```python
from build123d import *

# Parameters (mm, degrees)
BOSS_EXTRUDE1_DEPTH = 2.2
SKETCH2_W           = 9
SKETCH2_H           = 2.2
SKETCH2_W_2         = 42.2
BOSS_EXTRUDE2_DEPTH = 22.8
SKETCH3_W           = 9
SKETCH3_H           = 2.2
CUT_EXTRUDE1_DEPTH  = 50.796084183
SKETCH4_R           = 1.5
CUT_EXTRUDE2_DEPTH  = 54.851740919
SKETCH5_R           = 4
SKETCH5_R_2         = 1.5
CUT_EXTRUDE3_DEPTH  = 53.866340899


with BuildPart() as part:
    # Sketch1 → Boss-Extrude1 (new body)
    with BuildSketch(Plane(origin=(0, 0, 0), x_dir=(1, 0, 0), z_dir=(0, 1, 0))):
        Polygon((21.1, 0), (-21.1, 0), (-21.1, 8), (-30.1, 8), (-30.1, 33), (-21.1, 33), (-21.1, 27), (-18.1, 27), (-18.1, 37), (18.1, 37), (18.1, 27), (21.1, 27), (21.1, 33), (30.1, 33), (30.1, 8), (21.1, 8), align=None)
    extrude(amount=BOSS_EXTRUDE1_DEPTH)

    # Sketch2 → Boss-Extrude2 (add)
    with BuildSketch(Plane(origin=(0, 2.2, 0), x_dir=(1, 0, 0), z_dir=(0, 1, 0))):
        with Locations((25.6, 31.9)):
            Rectangle(SKETCH2_W, SKETCH2_H)
        with Locations((-25.6, 31.9)):
            Rectangle(SKETCH2_W, SKETCH2_H)
        with Locations((0, 1.1)):
            Rectangle(SKETCH2_W_2, SKETCH2_H)
    extrude(amount=BOSS_EXTRUDE2_DEPTH)

    # Sketch3 → Cut-Extrude1 (cut, through all)
    with BuildSketch(Plane.XY.offset(-30.8)):
        with Locations((-25.6, 23.9)):
            Rectangle(SKETCH3_W, SKETCH3_H)
    extrude(amount=-CUT_EXTRUDE1_DEPTH, mode=Mode.SUBTRACT)

    # Sketch4 → Cut-Extrude2 (cut, through all)
    with BuildSketch(Plane.XY):
        with Locations((-17.5, 13)):
            Circle(SKETCH4_R)
        with Locations((-10.5, 13)):
            Circle(SKETCH4_R)
        with Locations((-10.5, 20)):
            Circle(SKETCH4_R)
        with Locations((-3.5, 13)):
            Circle(SKETCH4_R)
        with Locations((-10.5, 6)):
            Circle(SKETCH4_R)
        with Locations((10.5, 6)):
            Circle(SKETCH4_R)
        with Locations((3.5, 13)):
            Circle(SKETCH4_R)
        with Locations((10.5, 20)):
            Circle(SKETCH4_R)
        with Locations((10.5, 13)):
            Circle(SKETCH4_R)
        with Locations((17.5, 13)):
            Circle(SKETCH4_R)
    extrude(amount=-CUT_EXTRUDE2_DEPTH, mode=Mode.SUBTRACT)

    # Sketch5 → Cut-Extrude3 (cut, through all)
    with BuildSketch(Plane(origin=(0, 2.2, 0), x_dir=(1, 0, 0), z_dir=(0, 1, 0))):
        with Locations(Location((-10.5, 24.5, 0), (0, 0, 270))):
            Circle(SKETCH5_R)
        with Locations(Location((-17.5, 24.5, 0), (0, 0, 270))):
            Circle(SKETCH5_R_2)
        with Locations(Location((-10.5, 31.5, 0), (0, 0, 270))):
            Circle(SKETCH5_R_2)
        with Locations(Location((-3.5, 24.5, 0), (0, 0, 270))):
            Circle(SKETCH5_R_2)
        with Locations(Location((-10.5, 17.5, 0), (0, 0, 270))):
            Circle(SKETCH5_R_2)
        with Locations(Location((10.5, 17.5, 0), (0, 0, 90))):
            Circle(SKETCH5_R_2)
        with Locations(Location((3.5, 24.5, 0), (0, 0, 90))):
            Circle(SKETCH5_R_2)
        with Locations(Location((10.5, 31.5, 0), (0, 0, 90))):
            Circle(SKETCH5_R_2)
        with Locations(Location((17.5, 24.5, 0), (0, 0, 90))):
            Circle(SKETCH5_R_2)
        with Locations(Location((10.5, 24.5, 0), (0, 0, 90))):
            Circle(SKETCH5_R)
    extrude(amount=-CUT_EXTRUDE3_DEPTH, mode=Mode.SUBTRACT)


solid = part.part
```
Build history of the part. All positions in model axes, mm. A direction names the side the tool comes from. Round coordinates to 2 decimals unless told otherwise and drop trailing zeros. Write each loop counter-clockwise with the first axis right and the second up, starting at its lowest first coordinate (ties: lowest second). Pieces come first, ordered by that corner, then holes.
1) Mould opens along X. For faces 1 (the flat face through (-30.1, 2, -25)), 2 (the cylindrical face through (10.43, 1.12, -16)), 3 (the flat face through (21.1, 10, -2)) say: +X half, -X half, draft (parallel to the pull), parting line (faces both ways), or undercut.
2) Band-saw the part on C-C, the plane y = 19.25. List the corners of the cut face in (x, z), and give its area (3 significant figures).
3) Band-saw the part on B-B, the plane z = -31.5. List the corners of the cut face in (x, y), and give its area (3 significant figures).
4) Band-saw the part on D-D, the plane z = -17. List the corners of the cut face in (x, y).
5) 3-axis set-ups, long thin cutter, end or side, ignore diameter. For faces 4 (the flat face through (26, 1, -8)), 5 (the flat face through (-26, 1, -8)), 6 (the flat face through (-26, 12, -30.8)): which of +Z, -Z, +X, -X, +Y, -Y reach the whole face in a straight line?
6) Band-saw the part on A-A, the plane x = -17.5. List the corners of the cut face in (y, z), and give its area (3 significant figures).
7) Pin check, flat tips, straight feed: pin 1 (6.5 mm diameter, centred on x = -10.5, z = -24.5, fed in from -Y); pin 2 (8 mm diameter, centred on x = -19, y = 18.5, fed in from -Z); pin 3 (3.5 mm diameter, centred on x = 3.5, y = 13, fed in from -Z); pin 4 (6.5 mm diameter, centred on y = 15, z = -3.5, fed in from -X). Stop position of each tip, or through.
8) Drill centre lines: probe 1 along Y at (x, z) = (10.5, -1.6); probe 2 along Z at (x, y) = (25.5, 11); probe 3 along Y at (x, z) = (21, -20.5). Where is each one in solid material? Low to high.
Ans:
1. face 1: -X half
1. face 2: undercut
1. face 3: +X half
2. outline: (-30.1, -33) - (-21.1, -33) - (-21.1, -30.8) - (-30.1, -30.8) - close; (-21.1, -2.2) - (-11.8, -2.2) - (-11.8, 0) - (-21.1, 0) - close; (-9.2, -2.2) - (9.2, -2.2) - (9.2, 0) - (-9.2, 0) - close; (11.8, -2.2) - (21.1, -2.2) - (21.1, 0) - (11.8, 0) - close; (21.1, -33) - (30.1, -33) - (30.1, -30.8) - (21.1, -30.8) - close
2. area: 121 mm2
3. outline: (-30.1, 0) - (-21.1, 0) - (-21.1, 22.8) - (-30.1, 22.8) - close; (-18.1, 0) - (-12, 0) - (-12, 2.2) - (-18.1, 2.2) - close; (-9, 0) - (9, 0) - (9, 2.2) - (-9, 2.2) - close; (12, 0) - (18.1, 0) - (18.1, 2.2) - (12, 2.2) - close; (21.1, 0) - (30.1, 0) - (30.1, 25) - (21.1, 25) - close
3. area: 497 mm2
4. outline: (-30.1, 0) - (-11.91, 0) - (-11.91, 2.2) - (-30.1, 2.2) - close; (-9.09, 0) - (9.09, 0) - (9.09, 2.2) - (-9.09, 2.2) - close; (11.91, 0) - (30.1, 0) - (30.1, 2.2) - (11.91, 2.2) - close
5. face 4: +Z, +X, +Y, -Y
5. face 5: +Z, -X, +Y, -Y
5. face 6: +Z, +X, -X, +Y
6. outline: (0, -37) - (2.2, -37) - (2.2, -26) - (0, -26) - close; (0, -23) - (2.2, -23) - (2.2, -2.2) - (11.5, -2.2) - (11.5, 0) - (0, 0) - close; (14.5, -2.2) - (25, -2.2) - (25, 0) - (14.5, 0) - close
6. area: 118 mm2
7. pin 1: passes through
7. pin 2: stops at z = -33
7. pin 3: stops at z = -2.2
7. pin 4: stops at x = -21.1
8. probe 1: y = 0 to 4.5, 7.5 to 11.5, 14.5 to 18.5, 21.5 to 25
8. probe 2: z = -33 to -30.8
8. probe 3: y = 0 to 2.2
